Verification items for the finished model (mm, model axes). A direction names the side the tool comes from. Give positions to 0.01 mm unless a question says otherwise; leave off trailing zeros. Write each loop counter-clockwise with the first axis right and the second up, starting at its lowest first coordinate (ties: lowest second). Pieces come first, ordered by that corner, then holes. Notation, with made-up numbers: (19, 23.25) - (35, 23.25) arc R16 ccw to (35, 27.25) - close; hole circle Ø6 at (-18.5, 84.25). An arc over 180 degrees is marked (long way). Put each result on its own line as item: value.
from build123d import *

# Parameters (mm, degrees)
SKETCH1_W           = 25
SKETCH1_H           = 25
BOSS_EXTRUDE1_DEPTH = 22.5
SKETCH4_W           = 25
SKETCH4_H           = 25
BOSS_EXTRUDE2_DEPTH = 20
CUT_EXTRUDE2_DEPTH  = 42.5
CUT_EXTRUDE3_DEPTH  = 21.5
SKETCH6_R           = 2.25
CUT_EXTRUDE4_DEPTH  = 10
SKETCH10_R          = 2.5
CUT_EXTRUDE7_DEPTH  = 10
CUT_EXTRUDE8_DEPTH  = 2.6
SKETCH8_W           = 45
SKETCH8_H           = 12.480087705
CUT_EXTRUDE9_DEPTH  = 50


with BuildPart() as part:
    # Sketch1 → Boss-Extrude1 (new, symmetric)
    with BuildSketch(Plane(origin=(0, 0, 0), x_dir=(1, 0, 0), z_dir=(0, 1, 0))):
        Rectangle(SKETCH1_W, SKETCH1_H)
    extrude(amount=BOSS_EXTRUDE1_DEPTH, both=True)

    # Sketch4 → Boss-Extrude2 (add)
    with BuildSketch(Plane.ZY.offset(12.5)):
        with Locations((0, 10)):
            Rectangle(SKETCH4_W, SKETCH4_H)
    extrude(amount=BOSS_EXTRUDE2_DEPTH)

    # Sketch3 → Cut-Extrude2 (cut)
    with BuildSketch(Plane.XZ.offset(22.5)):
        Polygon((-2.75, 4.5), (-2.75, 10), (-10.25, 10), (-10.25, 2.75), (-4.75, 2.75), (-4.75, -2.75), (-10.25, -2.75), (-10.25, -10.25), (-2.75, -10.25), (-2.75, -4.75), (2.75, -4.75), (2.75, -10.25), (10, -10.25), (10, -2.75), (4.5, -2.75), (4.5, 2.75), (10, 2.75), (10, 10), (2.75, 10), (2.75, 4.5), align=None)
    extrude(amount=-CUT_EXTRUDE2_DEPTH, mode=Mode.SUBTRACT)

    # Sketch5 → Cut-Extrude3 (cut)
    with BuildSketch(Plane.ZY.offset(32.5)):
        Polygon((-10.125, 7.25), (-10.125, -0.125), (-2.75, -0.125), (-2.75, 5.375), (2.75, 5.375), (2.75, -0.125), (10.125, -0.125), (10.125, 7.25), (4.625, 7.25), (4.625, 12.75), (10.125, 12.75), (10.125, 20.125), (2.75, 20.125), (2.75, 14.625), (-2.75, 14.625), (-2.75, 20.125), (-10.125, 20.125), (-10.125, 12.75), (-4.625, 12.75), (-4.625, 7.25), align=None)
    extrude(amount=-CUT_EXTRUDE3_DEPTH, mode=Mode.SUBTRACT)

    # Sketch6 → Cut-Extrude4 (cut)
    with BuildSketch(Plane(origin=(0, 0, -12.5), x_dir=(-1, 0, 0), z_dir=(0, 0, -1))):
        with Locations((0, -12.5)):
            Circle(SKETCH6_R)
        with Locations((22.5, 10)):
            Circle(SKETCH6_R)
    extrude(amount=-CUT_EXTRUDE4_DEPTH, mode=Mode.SUBTRACT)

    # Sketch10 → Cut-Extrude7 (cut)
    with BuildSketch(Plane.XY.offset(12.5)):
        with Locations((-27.5, 10)):
            Circle(SKETCH10_R)
        with Locations((0, -17.5)):
            Circle(SKETCH10_R)
    extrude(amount=-CUT_EXTRUDE7_DEPTH, mode=Mode.SUBTRACT)

    # Sketch11 → Cut-Extrude8 (cut)
    with BuildSketch(Plane(origin=(0, 0, 4.5), x_dir=(-1, 0, 0), z_dir=(0, 0, -1))):
        Polygon((2.222626661, -13.550219745), (-2.309296709, -13.600258721), (-4.53192337, -17.550038976), (-2.222626661, -21.449780255), (2.309296709, -21.399741279), (4.53192337, -17.449961024), align=None)
        Polygon((31.412394942, 12.287793512), (27.474910171, 14.532130165), (23.562515229, 12.244336654), (23.587605058, 7.712206488), (27.525089829, 5.467869835), (31.437484771, 7.755663346), align=None)
    extrude(amount=-CUT_EXTRUDE8_DEPTH, mode=Mode.SUBTRACT)

    # Sketch8 → Cut-Extrude9 (cut)
    with BuildSketch(Plane(origin=(0, 22.5, 0), x_dir=(1, 0, 0), z_dir=(0, 1, 0))):
        with Locations((-10, 6.259956147)):
            Rectangle(SKETCH8_W, SKETCH8_H)
    extrude(amount=-CUT_EXTRUDE9_DEPTH, mode=Mode.SUBTRACT)

    # Loft1: read off the stored shape, not the designer's step
    # Loft1: loft between two sections, ruled curve by curve
    loft1_from = [
        Edge.make_bspline([(-20, -2.5, 8.740043853), (-20.833333333, -2.5, 8.740043853), (-21.666666667, -2.5, 8.740043853), (-23.333333333, -2.5, 8.740043853), (-24.166666667, -2.5, 8.740043853), (-25, -2.5, 8.740043853)], [0, 0, 0, 0, 0.5, 0.5, 1, 1, 1, 1], 3),
        Edge.make_bspline([(-25, -2.5, 8.740043853), (-25, -2.5, 7.906710519), (-25, -2.5, 7.073377186), (-25, -2.5, 5.406710519), (-25, -2.5, 4.573377186), (-25, -2.5, 3.740043853)], [0, 0, 0, 0, 0.5, 0.5, 1, 1, 1, 1], 3),
        Edge.make_bspline([(-20, -2.5, 3.740043853), (-20, -2.5, 4.573377186), (-20, -2.5, 5.406710519), (-20, -2.5, 7.073377186), (-20, -2.5, 7.906710519), (-20, -2.5, 8.740043853)], [0, 0, 0, 0, 0.5, 0.5, 1, 1, 1, 1], 3),
        Edge.make_bspline([(-25, -2.5, 3.740043853), (-24.166666667, -2.5, 3.740043853), (-23.333333333, -2.5, 3.740043853), (-21.666666667, -2.5, 3.740043853), (-20.833333333, -2.5, 3.740043853), (-20, -2.5, 3.740043853)], [0, 0, 0, 0, 0.5, 0.5, 1, 1, 1, 1], 3),
    ]
    loft1_to = [
        Edge.make_bspline([(-12.5, -15, 8.740043853), (-12.5, -15, 7.906710519), (-12.5, -15, 7.073377186), (-12.5, -15, 5.406710519), (-12.5, -15, 4.573377186), (-12.5, -15, 3.740043853)], [0, 0, 0, 0, 0.5, 0.5, 1, 1, 1, 1], 3),
        Edge.make_bspline([(-12.5, -15, 3.740043853), (-12.5, -14.166666667, 3.740043853), (-12.5, -13.333333333, 3.740043853), (-12.5, -11.666666667, 3.740043853), (-12.5, -10.833333333, 3.740043853), (-12.5, -10, 3.740043853)], [0, 0, 0, 0, 0.5, 0.5, 1, 1, 1, 1], 3),
        Edge.make_bspline([(-12.5, -10, 8.740043853), (-12.5, -10.833333333, 8.740043853), (-12.5, -11.666666667, 8.740043853), (-12.5, -13.333333333, 8.740043853), (-12.5, -14.166666667, 8.740043853), (-12.5, -15, 8.740043853)], [0, 0, 0, 0, 0.5, 0.5, 1, 1, 1, 1], 3),
        Edge.make_bspline([(-12.5, -10, 3.740043853), (-12.5, -10, 4.573377186), (-12.5, -10, 5.406710519), (-12.5, -10, 7.073377186), (-12.5, -10, 7.906710519), (-12.5, -10, 8.740043853)], [0, 0, 0, 0, 0.5, 0.5, 1, 1, 1, 1], 3),
    ]
    loft1 = Solid(Shell([*[Face.make_surface_from_curves(loft1_from[k], loft1_to[k]) for k in range(4)], Face(Wire(loft1_from)), Face(Wire(loft1_to))]))
    add(loft1)


with BuildPart() as body_2:
    # Mirror1: mirrored copy
    add(part.part.mirror(Plane(origin=(0, 22.5, 0), x_dir=(0, 0, 1), z_dir=(0, -1, 0))))


solid = body_2.part
Q1. Set-up check for faces 1 (the face through (-32, 35, 4.625)), 2 (the face through (-22, 47.5, 3)), 3 (the face through (10, 47, 6)), 4 (the face through (-22, 29, 10.125)), 5 (the face through (-4.75, 47, 1)): record each of +Z, -Z, +X, -X, +Y, -Y from which the full face is reachable in a straight line by a thin tool's end or side.
Answers follow:
face 1: -Z, -X
face 2: none
face 3: +Y
face 4: -X
face 5: -Z, +Y
Q2. Go/stop test with flat-tipped pins: pin 1 Ø3.5 at (x, z) = (-19, 7.5) entering from +Y; pin 2 Ø6 at (x, y) = (0.5, 38) entering from -Z; pin 3 Ø6 at (x, y) = (-14.5, 35.5) entering from -Z (3 decimals). Record where each tip stops, or that it passes through.
Answers follow:
pin 1: stops at y = 54.5
pin 2: stops at z = 4.5
pin 3: stops at z = 4.625
Q3. Section check D-D, the plane x = -9.5. Record the cut outline in (y, z).
Answers follow:
outline: (22.5, -0.02) - (67.5, -0.02) - (67.5, 2.75) - (25, 2.75) - (25, 10) - (67.5, 10) - (67.5, 12.5) - (22.5, 12.5) - close
Q4. Section check C-C, the plane y = 62.5. Record the cut outline in (x, z).
Answers follow:
outline: (-12.5, -0.02) - (-4.75, -0.02) - (-4.75, 2.75) - (-10.25, 2.75) - (-10.25, 10) - (-2.75, 10) - (-2.75, 7.1) - (-2.5, 7.1) - (-2.5, 12.5) - (-12.5, 12.5) - close; (2.5, 7.1) - (2.75, 7.1) - (2.75, 10) - (10, 10) - (10, 2.75) - (4.5, 2.75) - (4.5, -0.02) - (12.5, -0.02) - (12.5, 12.5) - (2.5, 12.5) - close
Q5. Section check B-B, the plane x = -27.5. Record the cut outline in (y, z) (3 decimals).
Answers follow:
outline: (22.5, -0.02) - (30.375, -0.02) - (30.375, 2.75) - (24.875, 2.75) - (24.875, 10.125) - (32.25, 10.125) - (32.25, 7.1) - (32.5, 7.1) - (32.5, 12.5) - (22.5, 12.5) - close; (37.5, 7.1) - (37.75, 7.1) - (37.75, 10.125) - (45.125, 10.125) - (45.125, 2.75) - (39.625, 2.75) - (39.625, -0.02) - (47.5, -0.02) - (47.5, 12.5) - (37.5, 12.5) - close
Q6. Section check A-A, the plane y = 44. Record the cut outline in (x, z) (3 decimals), plus the area to 3 significant figures.
Answers follow:
outline: (-32.5, -0.02) - (-4.75, -0.02) - (-4.75, 2.75) - (-10.25, 2.75) - (-10.25, 10) - (-2.75, 10) - (-2.75, 4.5) - (2.75, 4.5) - (2.75, 10) - (10, 10) - (10, 2.75) - (4.5, 2.75) - (4.5, -0.02) - (12.5, -0.02) - (12.5, 12.5) - (-32.5, 12.5) - (-32.5, 10.125) - (-11, 10.125) - (-11, 2.75) - (-32.5, 2.75) - close
area: 263 mm2
Q7. Release check for a two-part mould opening along Y. For faces 6 (the face through (-10.25, 47, 6)), 7 (the face through (-10, 22.5, 6)), 8 (the face through (-22, 28, 2.75)) record: released by +Y, released by -Y, zero draft, split by the parting line, or undercut.
Answers follow:
face 6: zero draft
face 7: released by -Y
face 8: undercut
Q8. Scan lines: line 1 along X through (y, z) = (47, 8); line 2 along X through (y, z) = (35, 8.45); line 3 along Z through (x, y) = (-12.5, 27) (3 decimals). Record each from-to range of solid material in increasing order.
Answers follow:
line 1: x = -32.5 to -10.25, -2.75 to 2.75, 10 to 12.5
line 2: x = -32.5 to -30, -25 to -10.25, -2.75 to 2.75, 10 to 12.5
line 3: z = -0.02 to 2.75, 10.125 to 12.5
